Solid Edge part; units mm, degrees
sketch "Sketch1" plane through (0, 0, 0) normal (0, 0, 1) x (1, 0, 0)
  spline S0 degree 3 poles (-69.5242, 19.4932) (-23.3267, 12.9257) (22.6888, 12.9752) (68.6585, 19.674) knots 0 0 0 0 1 1 1 1
  spline S1 degree 3 poles (-69.54, -19.6556) (-23.1773, -15.4302) (23.2615, -15.4924) (69.7765, -19.8423) knots 0 0 0 0 1 1 1 1
  arc A0 (-69.54, -19.6556) -> (-69.5242, 19.4932) centre (-75.1666, -0.0789) cw
  arc A1 (68.6585, 19.674) -> (69.7765, -19.8423) centre (75.0403, 0.0806) cw
extrude "Protrusion1" add sketch "Sketch1" along normal blind 3
sketch "Sketch2" plane through (0.0555, 0.0806, 3) normal (0, 0, 1) x (1, 0, 0)
  circle A0 centre (83.5848, 0) radius 1
  circle A1 centre (55.6848, 0) radius 1
  line L0 (-58.5721, -6.5095) -> (-58.5721, 6.1905)
  line L1 (-58.5721, 6.1905) -> (-81.1721, 6.1905)
  line L2 (-81.1721, 6.1905) -> (-81.1721, -6.5095)
  line L3 (-81.1721, -6.5095) -> (-58.5721, -6.5095)
  circle A2 centre (-83.8221, -0.1595) radius 1
  circle A3 centre (-55.9221, -0.1595) radius 1
  line L4 (58.3348, 6.35) -> (58.3348, -6.35)
  line L5 (58.3348, -6.35) -> (80.9348, -6.35)
  line L6 (80.9348, -6.35) -> (80.9348, 6.35)
  line L7 (80.9348, 6.35) -> (58.3348, 6.35)
  dimension "D1" = 58.3348
  dimension "D2" = 58.3348
  dimension "D3" = 58.3348
extrude "ExtrudedCutout_1" cut sketch "Sketch2" against normal blind 484.752
sketch "Sketch3" plane through (0.0555, 0.0806, 3) normal (0, 0, 1) x (1, 0, 0)
  line L0 (29.6848, 27.4896) -> (-99.1539, 27.4896)
  line L1 (-99.1539, 27.4896) -> (-99.1539, -25.8213)
  line L2 (-99.1539, -25.8213) -> (29.6848, -25.8213)
  line L3 (29.6848, -25.8213) -> (29.6848, 27.4896)
extrude "ExtrudedCutout_2" cut sketch "Sketch3" against normal blind 169.5138
sketch "Sketch4" plane through (0, 0, 0) normal (0, 0, 1) x (1, 0, 0)
  line L0 (29.7403, -17.1563) -> (29.7403, 15.5915)
  spline S0 degree 3 poles (29.7403, 15.5915) (42.2697, 16.3768) (55.2702, 17.7412) (68.6585, 19.674) knots 0 0 0 0 1 1 1 1
  spline S1 degree 3 poles (29.7403, -17.1563) (34.3353, -17.3622) (40.0841, -17.6253) (48.6781, -18.1532) (57.9287, -18.805) (64.4454, -19.3301) (69.7765, -19.8423) knots 0 0 0 0 0.312805 0.467988 0.637686 1 1 1 1
  arc A0 (68.6585, 19.674) -> (69.7765, -19.8423) centre (75.0403, 0.0806) cw
  line L1 (58.3903, -6.2694) -> (58.3903, 6.4306)
  line L2 (58.3903, 6.4306) -> (80.9903, 6.4306)
  line L3 (80.9903, 6.4306) -> (80.9903, -6.2694)
  line L4 (80.9903, -6.2694) -> (58.3903, -6.2694)
  circle A1 centre (55.7403, 0.0806) radius 1
  circle A2 centre (83.6403, 0.0806) radius 1
  line L5 (29.7403, -17.1563) -> (29.7403, 15.5915)
  spline S2 degree 3 poles (29.7403, 15.5915) (17.2109, 16.3768) (4.2104, 17.7412) (-9.1779, 19.674) knots 0 0 0 0 1 1 1 1
  arc A3 (-9.1779, 19.674) -> (-10.2959, -19.8423) centre (-15.5597, 0.0806) ccw
  spline S3 degree 3 poles (29.7403, -17.1563) (25.1453, -17.3622) (19.3965, -17.6253) (10.8024, -18.1532) (1.5519, -18.805) (-4.9648, -19.3301) (-10.2959, -19.8423) knots 0 0 0 0 0.312805 0.467988 0.637686 1 1 1 1
  line L6 (1.0903, -6.2694) -> (1.0903, 6.4306)
  line L7 (1.0903, 6.4306) -> (-21.5097, 6.4306)
  line L8 (-21.5097, 6.4306) -> (-21.5097, -6.2694)
  line L9 (-21.5097, -6.2694) -> (1.0903, -6.2694)
  circle A4 centre (3.7403, 0.0806) radius 1
  circle A5 centre (-24.1597, 0.0806) radius 1
extrude "ExtrudedProtrusion_2" add sketch "Sketch4" against normal blind 3
sketch "Sketch5" plane through (-3.213, 0.0806, 0) normal (0, 0, 1) x (0, 1, 0)
  line L0 (25.6992, -32.9533) -> (-24.0131, -32.9533)
  line L1 (-24.0131, -32.9533) -> (-24.0131, 35.3247)
  line L2 (-24.0131, 35.3247) -> (25.6992, 35.3247)
  line L3 (25.6992, 35.3247) -> (25.6992, -32.9533)
extrude "ExtrudedCutout_3" cut sketch "Sketch5" against normal blind 310.7547
sketch "Sketch6" plane through (69.6903, 6.4306, 0) normal (0, -1, 0) x (1, 0, 0)
  line L0 (-39.95, 3) -> (25.9565, 3)
  line L1 (25.9565, 3) -> (25.9565, 0)
  line L2 (25.9565, 0) -> (-39.95, 0)
  line L3 (-39.95, 0) -> (-39.95, 3)
extrude "ExtrudedCutout_4" cut sketch "Sketch6" against normal blind 369.6121
sketch "Sketch7" plane through (69.6903, -6.2694, 0) normal (0, 1, 0) x (1, 0, 0)
  line L0 (-39.95, -0.4111) -> (-39.95, -3)
  line L1 (-39.95, -3) -> (25.7218, -3)
  line L2 (25.7218, -3) -> (25.9565, 0)
  line L3 (25.9565, 0) -> (-39.95, -0.4111)
extrude "ExtrudedCutout_5" cut sketch "Sketch7" against normal blind 176.465
sketch "Sketch8" plane through (29.7403, -0.7635, 0) normal (-1, 0, 0) x (0, -1, 0)
  line L0 (20.933, 0) -> (-7.194, 0)
  line L1 (-7.194, 0) -> (-7.194, 4.1468)
  line L2 (-7.194, 4.1468) -> (20.933, 4.1468)
  line L3 (20.933, 4.1468) -> (20.933, 0)
extrude "ExtrudedCutout_6" cut sketch "Sketch8" against normal blind 228.3963
sketch "Sketch9" plane through (0, 0, 0) normal (0, 0, 1) x (1, 0, 0)
  line L0 (-21.5097, -6.2694) -> (-21.5097, 6.4306)
  line L1 (-21.5097, 6.4306) -> (1.0903, 6.4306)
  line L2 (1.0903, -6.2694) -> (1.0903, 6.4306)
  line L3 (1.0903, -6.2694) -> (-21.5097, -6.2694)
  circle A0 centre (3.7403, 0.0806) radius 1
  circle A1 centre (-24.1597, 0.0806) radius 1
  spline S0 degree 3 poles (29.7403, 15.5915) (17.2977, 16.3681) (4.325, 17.7289) (-9.1779, 19.674) knots 0 0 0 0 1 1 1 1
  arc A2 (-9.1779, 19.674) -> (-10.2959, -19.8423) centre (-15.5597, 0.0806) ccw
  spline S1 degree 3 poles (29.7403, -17.1563) (17.4202, -17.6536) (4.1171, -18.5003) (-10.2959, -19.8423) knots 0 0 0 0 1 1 1 1
  line L4 (29.7403, -17.1563) -> (29.7403, 15.5915)
extrude "ExtrudedProtrusion_3" add sketch "Sketch9" against normal blind 3
sketch "Sketch10" plane through (29.7403, 0.0806, 0) normal (0, 0, 1) x (1, 0, 0)
  line L0 (-24.0106, -8.9531) -> (-56.723, -8.9531)
  line L1 (-56.723, -8.9531) -> (-56.723, 8.934)
  line L2 (-56.723, 8.934) -> (-24.0106, 8.934)
  line L3 (-24.0106, 8.934) -> (-24.0106, -8.9531)
  line L4 (23.0437, -9.1142) -> (23.0437, 9.5786)
  line L5 (23.0437, 9.5786) -> (56.723, 9.5786)
  line L6 (56.723, 9.5786) -> (56.723, -9.1142)
  line L7 (56.723, -9.1142) -> (23.0437, -9.1142)
extrude "ExtrudedProtrusion_4" add sketch "Sketch10" against normal blind 3
sketch "Sketch11" plane through (29.7403, 0.0806, 0) normal (0, 0, 1) x (1, 0, 0)
  circle A0 centre (-45.3, 0) radius 1.5
  circle A1 centre (45.3, 0) radius 1.5
  circle A2 centre (0, 0) radius 1.5
extrude "Cutout1" cut sketch "Sketch11" against normal blind 593.6896
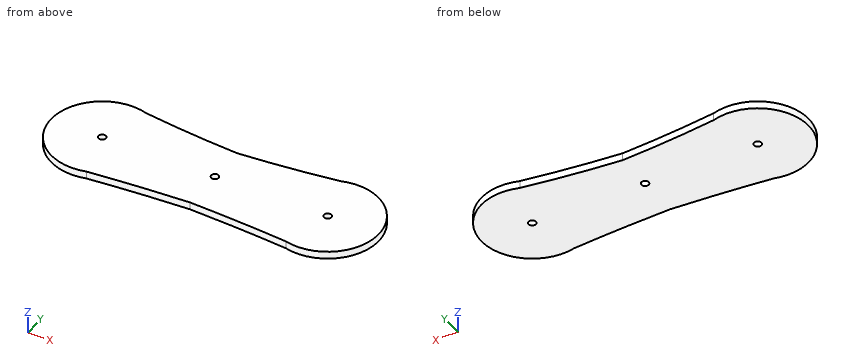
Here's how the part is built. I have some questions about the finished solid (model axes, mm). Give positions to 0.01 mm unless a question says otherwise; leave off trailing zeros. Loops run counter-clockwise (first coordinate to the right, second up) from the corner with the lowest first, then second, coordinate; pieces in that order, holes last. Notation, with made-up numbers: M 34,65.25 L 64,65.25 A6 cw 64,75.25 Z; hole C 64,-19.5 d9. An arc over 180 degrees is marked long. Put each result on its own line as item: value. Start each with the question number.
(1) I want a section at C-C on z = -1.8. State how many separate pieces and enclosed holes the cut face has, then the cut area to 3 significant figures.
(2) I want a section at B-B on x = -25.5. Please give me the cut outline in (y, z).
(3) I need wall thicknesses on line 1 along Y through (x, z) = (74, -2.7); line 2 along X through (y, z) = (-15, -0.6); line 3 along X through (y, z) = (10.5, -1.05). Which ranges of each line are inside material? Lowest first, please. Write a range as [from, to].
(4) I want a section at A-A on y = 8. Please give me the cut outline in (x, z).
Answer block:
1. separate pieces: 1
1. enclosed holes: 3
1. area: 4,610 mm^2
2. outline: M -17.97,-3 L 18.13,-3 L 18.13,0 L -17.97,0 Z
3. line 1: [-20.5, -1], [1.16, 20.66]
3. line 2: [-29.6, 89.08]
3. line 3: [-33.34, 92.82]
4. outline: M -34.58,-3 L 94.06,-3 L 94.06,0 L -34.58,0 Z
